Drawing for the job (mm, zero at the part's lowest x, y, z). A direction names the side the tool comes from. Coordinates: 2 decimals unless noted, no trailing zeros. Loops run counter-clockwise (first coordinate to the right, second up) from the corner with the lowest first, then second, coordinate; pieces in that order, holes last.
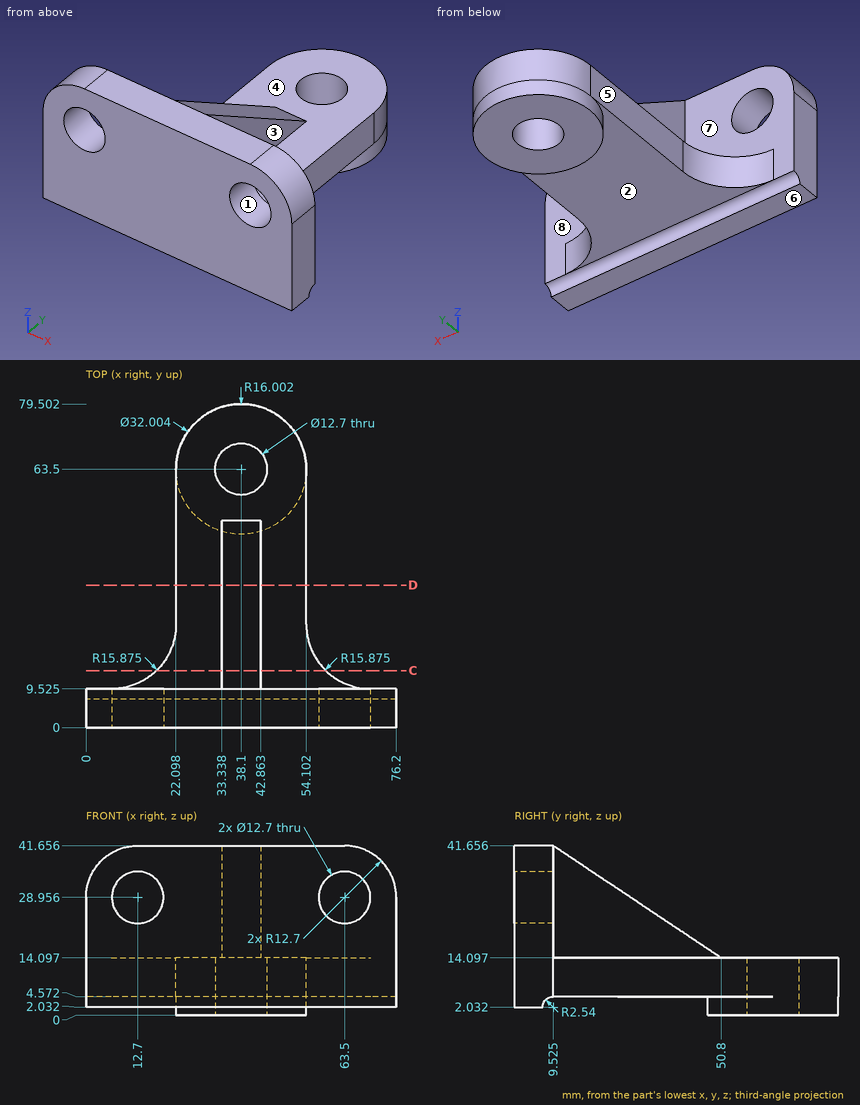
Q1. Saw through at C-C (y = 14). List the corners of the cut face in (x, z).
Q2. Tool access for the marked faces 4, 5, 6, 7 and 8: list every direction of +Z, -Z, +X, -X, +Y, -Y with a clear straight run to the whole face (end or side of a thin tool).
Q3. Probe line 1 (X direction, y = 63, z = 10); line 2 (Y direction, x = 38, z = 6); line 3 (X direction, y = 14, z = 38). List the from-to ranges inside material, lowest first.
Q4. Mould opens along X. For the marked faces 1, 2 and 3 say: released by +X, released by -X, zero draft, split by the parting line, or undercut.
Q5. Saw through at D-D (y = 35). List the corners of the cut face in (x, z), plus the area to 3 significant figures.
Q6. Drop flat-ended pins along their axis: P1, Ø7.5, axis at y = 45, z = 11.5, coming from the +X side; P2, Ø14, axis at y = 24.5, z = 21.5, coming from the -X side; P3, Ø12, axis at x = 17.5, y = 70.5, coming from the +Z side; P4, Ø11.5, axis at x = 63.5, z = 28.956, coming from the +Y side. Give the stop position or say it passes through.
Checked values:
1. outline: (17.27, 4.57) - (58.93, 4.57) - (58.93, 14.1) - (42.86, 14.1) - (42.86, 38.67) - (33.34, 38.67) - (33.34, 14.1) - (17.27, 14.1) - close
2. face 4: +Z, +Y
2. face 5: +Z, -Z, -X, +Y
2. face 6: -Z, +X, -X, -Y
2. face 7: +Z, -X, +Y
2. face 8: +Z, +X, +Y
3. line 1: x = 22.1 to 31.77, 44.43 to 54.1
3. line 2: y = 0 to 57.15, 69.85 to 79.5
3. line 3: x = 33.34 to 42.86
4. face 1: undercut
4. face 2: zero draft
4. face 3: released by +X
5. outline: (22.1, 4.57) - (54.1, 4.57) - (54.1, 14.1) - (42.86, 14.1) - (42.86, 24.65) - (33.34, 24.65) - (33.34, 14.1) - (22.1, 14.1) - close
5. area: 405 mm2
6. P1: stops at x = 54.1
6. P2: stops at x = 33.34
6. P3: stops at z = 14.1
6. P4: passes through
